Autodesk Inventor part; units mm, degrees
ref_plane "作業平面1" through (-124.0859, 3.5, -124.0859) normal (0, 1, 0) x (0.0824, 0, 0.9966)
ref_plane "YZ Plane" through (0, 0, 0) normal (1, 0, 0) x (0, 1, 0)
ref_plane "XZ Plane" through (0, 0, 0) normal (0, 1, 0) x (-1, 0, 0)
sketch "スケッチ1" plane through (0, 0, 0) normal (0, 1, 0) x (-1, 0, 0)
  circle A0 centre (0, 0) radius 42.5
  dimension "d0" = 85
extrude "押し出し1" add sketch "スケッチ1" along normal blind 1
sketch "スケッチ2" plane through (0, 0, 0) normal (0, -1, 0) x (1, 0, 0)
  circle A0 centre (-27.4257, 32.3702) radius 1.3
  circle A1 centre (32.3702, 27.4257) radius 1.3
  circle A2 centre (27.4257, -32.3702) radius 1.3
  circle A3 centre (-32.3702, -27.4257) radius 1.3
  circle A4 centre (-32.3702, -27.4257) radius 4
  circle A5 centre (-27.4257, 32.3702) radius 4
  circle A6 centre (27.4257, -32.3702) radius 4
  circle A7 centre (32.3702, 27.4257) radius 4
  circle A8 centre (-13, 39.5) radius 1.35
  circle A9 centre (39.5, 13) radius 1.35
  circle A10 centre (13, -39.5) radius 1.35
  circle A11 centre (-39.5, -13) radius 1.35
  circle A12 centre (-39.5, -13) radius 4
  circle A13 centre (-13, 39.5) radius 4
  circle A14 centre (39.5, 13) radius 4
  circle A15 centre (13, -39.5) radius 4
  line L0 (17.7859, 38.8061) -> (-24.7141, -34.8061)
  line L1 (-24.7141, -34.8061) -> (-17.7859, -38.8061)
  line L2 (-17.7859, -38.8061) -> (24.7141, 34.8061)
  line L3 (24.7141, 34.8061) -> (17.7859, 38.8061)
  line L4 (17.7859, 38.8061) -> (-17.7859, -38.8061) construction
  line L5 (-24.7141, -34.8061) -> (24.7141, 34.8061) construction
  line L6 (17.7859, -38.8061) -> (-24.7141, 34.8061)
  line L7 (-24.7141, 34.8061) -> (-17.7859, 38.8061)
  line L8 (-17.7859, 38.8061) -> (24.7141, -34.8061)
  line L9 (24.7141, -34.8061) -> (17.7859, -38.8061)
  line L10 (17.7859, -38.8061) -> (-17.7859, 38.8061) construction
  line L11 (-24.7141, 34.8061) -> (24.7141, -34.8061) construction
  line L12 (42.5, -4) -> (-42.5, -4)
  line L13 (-42.5, -4) -> (-42.5, 4)
  line L14 (-42.5, 4) -> (42.5, 4)
  line L15 (42.5, 4) -> (42.5, -4)
  line L16 (42.5, -4) -> (-42.5, 4) construction
  line L17 (-42.5, -4) -> (42.5, 4) construction
  line L18 (-42.5, 24.5374) -> (0, 49.0748) construction
  line L19 (0, 49.0748) -> (42.5, 24.5374) construction
  line L20 (42.5, 24.5374) -> (42.5, -24.5374) construction
  line L21 (42.5, -24.5374) -> (0, -49.0748) construction
  line L22 (0, -49.0748) -> (-42.5, -24.5374) construction
  line L23 (-42.5, -24.5374) -> (-42.5, 24.5374) construction
  circle A16 centre (0, 0) radius 42.5
  circle A17 centre (0, 0) radius 30.5
  point P0 (-11.6542, -28.1856)
  point P1 (11.6542, -28.1856)
  point P2 (0, -8)
  point P3 (18.5824, -24.1856)
  point P4 (30.2366, -4)
  point P5 (6.9282, -4)
  point P6 (30.2366, 4)
  point P7 (18.5824, 24.1856)
  point P8 (6.9282, 4)
  point P9 (11.6542, 28.1856)
  point P10 (-11.6542, 28.1856)
  point P11 (0, 8)
  point P12 (-18.5824, 24.1856)
  point P13 (-30.2366, 4)
  point P14 (-6.9282, 4)
  point P15 (-30.2366, -4)
  point P16 (-18.5824, -24.1856)
  point P17 (-6.9282, -4)
  point P18 (-26.4694, 33.2509)
  point P19 (-28.4514, 31.5716)
  point P20 (-33.2509, -26.4694)
  point P21 (-31.5716, -28.4514)
  dimension "d3" = 8
  dimension "d6" = 8
  dimension "d7" = 12
extrude "押し出し2" cut sketch "スケッチ2" against normal through all contours A0 A16 | L6 L14 A17 | A17 L0 L8 | L12 L0 A17 | A16 A8 A13 | A13 A16 A8 | A16 A11 A12 | A12 A16 A11 | A17 L14 L2 | A16 A8 | A8 A16 | L2 L6 A17 | A16 A11 | A11 A16 | L12 A17 L8 | A16 A3 | A16 A10 A15 | A15 A16 A10 | A16 A1 | A1 A16 | A16 A9 A14 | A14 A16 A9 | A16 A10 | A10 A16 | A16 A9 | A9 A16 | A16 A2 | A2 A16 picked at (-27.1376, 32.113) picked at (-32.0736, -27.1791)
sketch "スケッチ3" plane through (0, 0, 0) normal (0, -1, 0) x (1, 0, 0)
  arc A0 (-31.5716, -28.4514) -> (-33.2509, -26.4694) centre (-32.3702, -27.4257) ccw
  arc A1 (-28.4514, 31.5716) -> (-26.4694, 33.2509) centre (-27.4257, 32.3702) ccw
  arc A2 (31.5716, 28.4514) -> (33.2509, 26.4694) centre (32.3702, 27.4257) ccw
  arc A3 (28.4514, -31.5716) -> (26.4694, -33.2509) centre (27.4257, -32.3702) ccw
  circle A4 centre (-32.3702, -27.4257) radius 1.3
  circle A5 centre (-27.4257, 32.3702) radius 1.3
  circle A6 centre (32.3702, 27.4257) radius 1.3
  circle A7 centre (27.4257, -32.3702) radius 1.3
  circle A8 centre (-32.3702, -27.4257) radius 4
  circle A9 centre (-27.4257, 32.3702) radius 4
  circle A10 centre (32.3702, 27.4257) radius 4
  circle A11 centre (27.4257, -32.3702) radius 4
  point P0 (0, 0)
  point P1 (28.4514, -31.5716)
  point P2 (-26.4694, 33.2509)
  dimension "d10" = 8
ref_plane "作業平面1" through (-124.0859, 3.5, -124.0859) normal (0, 1, 0) x (0.0824, 0, 0.9966)
extrude "押し出し3" add sketch "スケッチ3" against normal up to surface (1 mm away)
properties part number "battery_cover"
The listing builds one solid part. Answer for the finished solid, in the listing's coordinates (mm). A direction names the side the tool comes from. Coordinates: 2 decimals unless noted, no trailing zeros. Loops run counter-clockwise (first coordinate to the right, second up) from the corner with the lowest first, then second, coordinate; pieces in that order, holes last. Notation, with made-up numbers: M -2.75,-3.75 L 32.25,-3.75 A17 ccw 32.25,25.25 Z; hole C 52,86.25 d2. An arc over 180 degrees is marked long. Answer as a JSON object with one key per item and string values. Group by question number.
Item 1: Determine the mould class of faces 5 (the face through (1, 1, 1)), 6 (the face through (-26.78, 0.49, 33.5)), 7 (the face through (20.68, 0.49, -37.13)), 8 (the face through (40.83, 0.49, -11.79)) for opening direction X: +X half, -X half, draft (parallel to the pull), parting line (faces both ways), or undercut.
Item 2: Section D-D (y = 0.25) is taken. Give the number of separate pieces and of enclosed holes in the cut face, and give its area (3 significant figures).
Item 3: Section B-B (z = 6.5) is taken. Write down the section's boundary in (x, y).
Item 4: Each of these flat-tipped pins is pushed along its axis until it touches: P1, Ø0.5, axis at x = 14, y = 0.5, coming from the -Z side; P2, Ø0.5, axis at x = -13, y = 0.5, coming from the -Z side. Where does it stop, or does it pass through?
Item 5: Section C-C (z = -13) is taken. Write down the section's boundary in (x, y), and give its area (3 significant figures).
Item 6: Section A-A (x = 13) is taken. Write down the section's boundary in (y, z), and give its area (3 significant figures).
Item 7: Consider L1, parallel to X at y = 0.45, z = 13; L2, parallel to Z at x = -21, y = 0.8; L3, parallel to X at y = 0.55, z = -13. Determine where each line is inside the solid, lowest interval first.
Item 8: Which of the six approach directions +Z, -Z, +X, -X, +Y, -Y give full straight-line access (tool end or side, diameter ignored) to faces 1 (the face through (-20.68, 0.49, 37.13)), 2 (the face through (-12.7, 0.5, -14)), 3 (the face through (-11.79, 0.49, -40.83)), 4 (the face through (37.13, 0.49, 20.68))?
Solved:
{
 "1": {"face 5": "draft", "face 6": "undercut", "face 7": "undercut", "face 8": "+X half"},
 "2": {"separate pieces": "1", "enclosed holes": "10", "area": "4,000 mm2"},
 "3": {"outline": "M -42,0 L -29.8,0 L -29.8,1 L -42,1 Z; M -8.37,0 L 8.37,0 L 8.37,1 L -8.37,1 Z; M 29.8,0 L 42,0 L 42,1 L 29.8,1 Z"},
 "4": {"P1": "stops at z = -35.7", "P2": "stops at z = -40.54"},
 "5": {"outline": "M -35.5,0 L -27.59,0 L -27.59,1 L -35.5,1 Z; M -12.12,0 L -2.89,0 L -2.89,1 L -12.12,1 Z; M 2.89,0 L 12.12,0 L 12.12,1 L 2.89,1 Z; M 27.59,0 L 40.46,0 L 40.46,1 L 27.59,1 Z", "area": "39.3 mm2"},
 "6": {"outline": "M 0,-35.5 L 1,-35.5 L 1,-14.52 L 0,-14.52 Z; M 0,-4 L 1,-4 L 1,4 L 0,4 Z; M 0,14.52 L 1,14.52 L 1,40.46 L 0,40.46 Z", "area": "54.9 mm2"},
 "7": {"L1": "x = -40.46 to -27.59, -12.12 to -2.89, 2.89 to 12.12, 27.59 to 35.5", "L2": "z = -36.95 to -22.12, -4 to 4, 22.12 to 36.95", "L3": "x = -35.5 to -27.59, -12.12 to -2.89, 2.89 to 12.12, 27.59 to 40.46"},
 "8": {"face 1": "+Z, +Y, -Y", "face 2": "+Y, -Y", "face 3": "-Z, +Y, -Y", "face 4": "+X, +Y, -Y"}
}
